Verification items for this drawing (mm, ordinates from the low corner). A direction names the side the tool comes from. Round coordinates to 2 decimals unless told otherwise and drop trailing zeros. Order: outer loops, then holes, each group sorted by start corner. A loop starts at its lowest first (then second) coordinate and runs counter-clockwise, first axis right, second up. Notation, with made-up numbers: (23, 78) - (50, 78) arc R14 ccw to (50, 85) - close; hole circle Ø1 at (14, -30). An arc over 180 degrees is marked (long way). Return JSON: item names as keys, results as strings. Group by question number.
Q1. Draft check along X on the marked faces 4, 5 and 6. Enter one of: pulls with the +X half, pulls with the -X half, needs draft (parallel to the pull), parting line crosses it, or undercut.
Q2. Sectioned sample at B-B, the plane x = 15. Record the cut outline in (y, z) (3 decimals), then the cut area to 3 significant figures.
Q3. Tool access check on the marked faces 1, 2 and 3. Record the directions out of +Z, -Z, +X, -X, +Y, -Y that give a thin tool (end or side, any length) a straight path to the whole face; none if there is none.
Q4. Material ranges on line 1 along X through (y, z) = (6.75, 15) (3 decimals); line 2 along X through (y, z) = (1.25, 13.25) (3 decimals), recorded low to high.
Q5. Sectioned sample at A-A, the plane z = 12.25. Record the cut outline in (x, y) (3 decimals).
Q6. Gauge pin test, flat ends, axial feed: pin 1 Ø6 at (x, z) = (13.5, 25) entering from -Y; pin 2 Ø4 at (y, z) = (8, 9) entering from +X (3 decimals); pin 3 Ø4.5 at (x, y) = (14, 8) entering from +Z (3 decimals); pin 4 Ø3 at (x, y) = (16.5, 7) entering from -Z (3 decimals). Record the tip position at first contact, or that the pin passes through.
Q7. Sectioned sample at C-C, the plane y = 1.5. Record the cut outline in (x, z) (3 decimals).
Q8. Sectioned sample at D-D, the plane x = 6.75. Record the cut outline in (y, z).
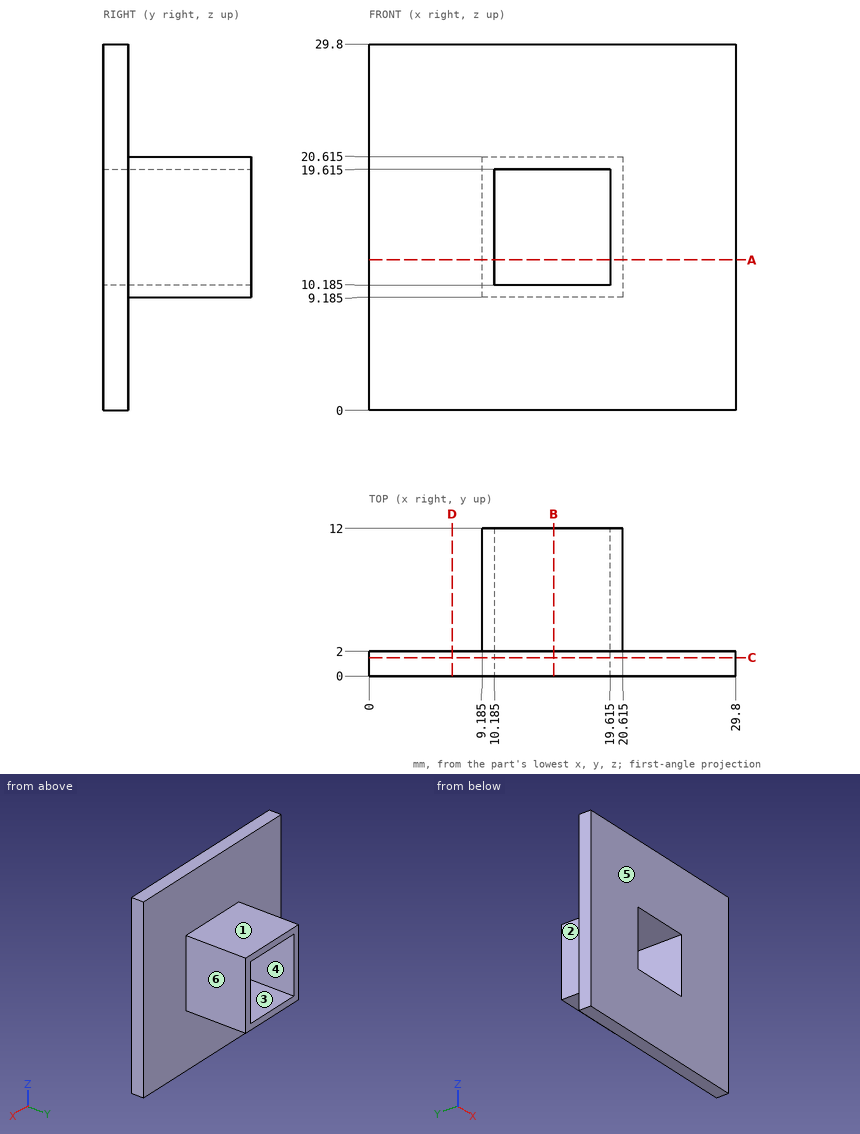
Reply:
{
 "1": {"face 4": "undercut", "face 5": "needs draft", "face 6": "pulls with the +X half"},
 "2": {"outline": "(0, 0) - (2, 0) - (2, 9.185) - (12, 9.185) - (12, 10.185) - (0, 10.185) - close; (0, 19.615) - (12, 19.615) - (12, 20.615) - (2, 20.615) - (2, 29.8) - (0, 29.8) - close", "area": "60.7 mm^2"},
 "3": {"face 1": "+Z, +X, -X, +Y", "face 2": "+Z, -Z, -X, +Y", "face 3": "+Y, -Y"},
 "4": {"line 1": "9.185 to 10.185, 19.615 to 20.615", "line 2": "0 to 10.185, 19.615 to 29.8"},
 "5": {"outline": "(0, 0) - (10.185, 0) - (10.185, 12) - (9.185, 12) - (9.185, 2) - (0, 2) - close; (19.615, 0) - (29.8, 0) - (29.8, 2) - (20.615, 2) - (20.615, 12) - (19.615, 12) - close"},
 "6": {"pin 1": "y = 0", "pin 2": "x = 20.615", "pin 3": "z = 20.615", "pin 4": "z = 9.185"},
 "7": {"outline": "(0, 0) - (29.8, 0) - (29.8, 29.8) - (0, 29.8) - close; hole (10.185, 10.185) - (19.615, 10.185) - (19.615, 19.615) - (10.185, 19.615) - close"},
 "8": {"outline": "(0, 0) - (2, 0) - (2, 29.8) - (0, 29.8) - close"}
}
